```python
from build123d import *

# Parameters (mm, degrees)
SKETCH1_R               = 15
BOSS_EXTRUDE1_DEPTH     = 680
SKETCH2_R               = 13.5
CUT_EXTRUDE1_DEPTH      = 681.33080189
CUT_EXTRUDE2_DEPTH      = 681.33080189
CUT_EXTRUDE2_DEPTH_BACK = 681.33080189
SKETCH3_R               = 1.5


with BuildPart() as part:
    # Sketch1 → Boss-Extrude1 (new body)
    with BuildSketch(Plane.XY):
        Circle(SKETCH1_R)
    extrude(amount=BOSS_EXTRUDE1_DEPTH)

    # Sketch2 → Cut-Extrude1 (cut, through all)
    with BuildSketch(Plane(origin=(0, 0, 0), x_dir=(-1, 0, 0), z_dir=(0, 0, -1))):
        Circle(SKETCH2_R)
    extrude(amount=-CUT_EXTRUDE1_DEPTH, mode=Mode.SUBTRACT)

    # Sketch3 → Cut-Extrude2 (cut, two sides: drawn at the far end of the back side and taken through both)
    with BuildSketch(Plane(origin=(0, 0, 0), x_dir=(1, 0, 0), z_dir=(0, 1, 0)).offset(-CUT_EXTRUDE2_DEPTH_BACK)):
        with Locations(Location((0, -15, 0), (0, 0, 270))):
            Circle(SKETCH3_R)
        with Locations(Location((0, -665, 0), (0, 0, 270))):
            Circle(SKETCH3_R)
        with Locations(Location((0, -79, 0), (0, 0, 270))):
            Circle(SKETCH3_R)
        with Locations(Location((0, -601, 0), (0, 0, 270))):
            Circle(SKETCH3_R)
    extrude(amount=CUT_EXTRUDE2_DEPTH + CUT_EXTRUDE2_DEPTH_BACK, mode=Mode.SUBTRACT)


solid = part.part
```
Here's how the part is built. I have some questions about the finished solid (model axes, mm). Round coordinates to 2 decimals unless told otherwise and drop trailing zeros. Loops run counter-clockwise (first coordinate to the right, second up) from the corner with the lowest first, then second, coordinate; pieces in that order, holes last. Notation, with made-up numbers: (41, 24) -> (50, 24) arc R18 ccw to (50, 38) -> close; hole circle Ø1 at (35, 35). An arc over 180 degrees is marked (long way). Answer as CSV lines item,"result".
1. If we section it at B-B on x = 9: Please give me the cut outline in (y, z).
Final values:
outline,"(-12, 0) -> (-10.06, 0) -> (-10.06, 680) -> (-12, 680) -> close; (10.06, 0) -> (12, 0) -> (12, 680) -> (10.06, 680) -> close"
2. If I drill on L1, parallel to Z at x = 0, y = -13.8; L2, parallel to X at y = -0.5, z = 248, over which ranges is the centre line in solid material (lowest first)?
Final values:
L1,"z = 0 to 13.5, 16.5 to 77.5, 80.5 to 599.5, 602.5 to 663.5, 666.5 to 680"
L2,"x = -14.99 to -13.49, 13.49 to 14.99"
3. If we section it at A-A on y = 0: Please give me the cut outline in (x, z).
Final values:
outline,"(-15, 0) -> (-13.5, 0) -> (-13.5, 680) -> (-15, 680) -> close; (13.5, 0) -> (15, 0) -> (15, 680) -> (13.5, 680) -> close"
4. For pin 1 (6 mm diameter, centred on y = 2.5, z = 221.5, fed in from +X); pin 2 (2 mm diameter, centred on y = -12, z = 543.5, fed in from +X); pin 3 (6 mm diameter, centred on x = 11.5, z = 533, fed in from +Y); pin 4 (1.5 mm diameter, centred on y = 6, z = 281.5, fed in from +X), each with a flat end and sliding along its axis, tell me the tip position at first contact or that it passes through.
Final values:
pin 1,"stops at x = 15"
pin 2,"stops at x = 10.2"
pin 3,"stops at y = 12.36"
pin 4,"stops at x = 14.05"
5. If we section it at C-C on z = 108: Please give me the cut outline in (x, y).
Final values:
outline,"circle Ø30 at (0, 0); hole circle Ø27 at (0, 0)"
6. Thinking about a two-plate mould opening in Y: for faces 1 (the face through (-14.985, 0.66, 335.24)), 2 (the face through (-11.18, 7.85, 680)), 3 (the face through (2.93, -13.18, 335.24)), which applies, released by +Y, released by -Y, zero draft, split by the parting line, or undercut?
Final values:
face 1,"split by the parting line"
face 2,"zero draft"
face 3,"undercut"
